Can you work these out from the model? Positions are in its coordinate system, mm. A direction names the side the tool comes from. Give positions to 0.01 mm unless a question says otherwise; leave off trailing zeros. Write each loop counter-clockwise with the first axis right and the second up, starting at its lowest first coordinate (ties: lowest second). Pieces come first, ordered by that corner, then holes.
from build123d import *

# Parameters (mm, degrees)
F0_R     = 1.55
F1_DEPTH = 5
F3_DEPTH = 165
F4_DEPTH = 25
F5_R     = 2.6
F6_DEPTH = 165.001


with BuildPart() as f1:
    # F0 (on Top) → F1 (new body)
    with BuildSketch(Plane.XY):
        Polygon((-10, -25), (10, -25), (10, -20), (10, 20), (10, 25), (-10, 25), (-10, 20), (-10, -20), align=None)
        with Locations((0, -10)):
            Circle(F0_R, mode=Mode.SUBTRACT)
        with Locations((0, 5)):
            Circle(F0_R, mode=Mode.SUBTRACT)
        Polygon((10, -20), (10, -25), (47.5, -55.5555555556), (47.5, -50.5555555556), align=None)
        Polygon((-47.5, -55.5555555556), (-10, -25), (-10, -20), (-47.5, -50.5555555556), align=None)
        Polygon((52.5, -59.6296296296), (47.5, -55.5555555556), (47.5, -95), (52.5, -95), align=None)
        Polygon((47.5, -50.5555555556), (47.5, -55.5555555556), (52.5, -59.6296296296), (52.5, -54.6296296296), align=None)
        Polygon((-52.5, -59.6296296296), (-47.5, -55.5555555556), (-47.5, -50.5555555556), (-52.5, -54.6296296296), align=None)
        Polygon((-47.5, -95), (-47.5, -55.5555555556), (-52.5, -59.6296296296), (-52.5, -95), align=None)
        Polygon((10, 25), (10, 20), (47.5, 50.5555555556), (47.5, 55.5555555556), align=None)
        Polygon((52.5, -54.6296296296), (52.5, -59.6296296296), (77.5, -80), (77.5, -75), align=None)
        Polygon((-47.5, 50.5555555556), (-10, 20), (-10, 25), (-47.5, 55.5555555556), align=None)
        Polygon((-77.5, -80), (-52.5, -59.6296296296), (-52.5, -54.6296296296), (-77.5, -75), align=None)
        Polygon((47.5, 55.5555555556), (47.5, 50.5555555556), (52.5, 54.6296296296), (52.5, 59.6296296296), align=None)
        Polygon((77.5, -75), (77.5, -80), (77.5, -95), (82.5, -95), (82.5, 95), (77.5, 95), (77.5, 80), (77.5, 75), align=None)
        Polygon((-52.5, 54.6296296296), (-47.5, 50.5555555556), (-47.5, 55.5555555556), (-52.5, 59.6296296296), align=None)
        Polygon((-77.5, -95), (-77.5, -80), (-77.5, -75), (-77.5, 75), (-77.5, 80), (-77.5, 95), (-82.5, 95), (-82.5, -95), align=None)
        Polygon((47.5, 95), (47.5, 55.5555555556), (52.5, 59.6296296296), (52.5, 95), align=None)
        Polygon((52.5, 59.6296296296), (52.5, 54.6296296296), (77.5, 75), (77.5, 80), align=None)
        Polygon((-52.5, 59.6296296296), (-47.5, 55.5555555556), (-47.5, 95), (-52.5, 95), align=None)
        Polygon((-77.5, 75), (-52.5, 54.6296296296), (-52.5, 59.6296296296), (-77.5, 80), align=None)
        Polygon((-52.5, -54.6296296296), (-47.5, -50.5555555556), (-47.5, 50.5555555556), (-52.5, 54.6296296296), align=None)
        Polygon((47.5, 50.5555555556), (47.5, -50.5555555556), (52.5, -54.6296296296), (52.5, 54.6296296296), align=None)
    extrude(amount=F1_DEPTH)

    # F2 (on face) → F3 (join, through all)
    with BuildSketch(Plane(origin=(-82.5, 0, 0), x_dir=(0, -1, 0), z_dir=(-1, 0, 0))):
        with BuildLine():
            Line((-95, 5), (-80, 5))
            ThreePointArc((-80, 5), (-87.5, 12.5), (-95, 5))
        make_face()
        with BuildLine():
            Line((80, 5), (95, 5))
            ThreePointArc((95, 5), (87.5, 12.5), (80, 5))
        make_face()
    extrude(amount=-F3_DEPTH)

    # F4 (cut): faces of the model
    f4_faces = [f1.faces().sort_by_distance(p)[0] for p in [
        (65, 87.5, 5),
        (0, 87.5, 5),
        (-65, 87.5, 5),
        (-65, -87.5, 5),
        (0, -87.5, 5),
        (65, -87.5, 5),
    ]]
    extrude(f4_faces, amount=-F4_DEPTH, mode=Mode.SUBTRACT)

    # F5 (on face) → F6 (cut, through all)
    with BuildSketch(Plane.YZ.offset(82.5)):
        with Locations((-87.5, 5)):
            Circle(F5_R)
        with Locations((87.5, 5)):
            Circle(F5_R)
    extrude(amount=-F6_DEPTH, mode=Mode.SUBTRACT)


solid = f1.part
(1) Imagine slicing it at D-D, the plane x = -23. Write out the boundary of the cut face in (y, z).
Returned:
outline: (-35.59, 0) - (-30.59, 0) - (-30.59, 5) - (-35.59, 5) - close; (30.59, 0) - (35.59, 0) - (35.59, 5) - (30.59, 5) - close
(2) If I drill on L1, parallel to Z at x = 81, y = -87; L2, parallel to X at y = 50, z = 2; L3, parallel to X at y = 47, z = 1, over which ranges is the centre line in solid material (lowest first)?
Returned:
L1: z = 0 to 2.45, 7.55 to 12.48
L2: x = -82.5 to -77.5, -52.5 to -47.5, -46.82 to -40.68, 40.68 to 46.82, 47.5 to 52.5, 77.5 to 82.5
L3: x = -82.5 to -77.5, -52.5 to -47.5, -43.14 to -37, 37 to 43.14, 47.5 to 52.5, 77.5 to 82.5
(3) For faces 4 (the face through (-64.82, 69.67, 2.46)), 5 (the face through (64.82, -69.67, 2.46)), 6 (the face through (77.5, 1, 2)), which set-ups out of +Z, -Z, +X, -X, +Y, -Y let a thin tool reach every point of the face, with its end or its side?
Returned:
face 4: +Z, -Z, +Y
face 5: +Z, -Z, -Y
face 6: +Z, -Z
(4) Will these pins go through, and if not, where does the flat tip stop? P1, Ø6, axis at x = -10.5, y = -32.5, coming from the -Z side; P2, Ø4, axis at x = 13.5, z = 2.5, coming from the -Y side; P3, Ø6, axis at y = 89, z = 3, coming from the +X side; P4, Ø6, axis at x = 29.5, z = 1.5, coming from the -Y side.
Returned:
P1: passes through
P2: stops at y = -29.48
P3: stops at x = 82.5
P4: stops at y = -43.33
(5) Imagine slicing it at A-A, the plane y = 87.5. Give the number of separate pieces and of enclosed holes in the cut face, plus the area to 3 significant figures.
Returned:
separate pieces: 8
enclosed holes: 0
area: 146 mm2
(6) Imagine slicing it at C-C, the plane y = -3.5. Write out the boundary of the cut face in (x, z).
Returned:
outline: (-82.5, 0) - (-77.5, 0) - (-77.5, 5) - (-82.5, 5) - close; (-52.5, 0) - (-47.5, 0) - (-47.5, 5) - (-52.5, 5) - close; (-10, 0) - (10, 0) - (10, 5) - (-10, 5) - close; (47.5, 0) - (52.5, 0) - (52.5, 5) - (47.5, 5) - close; (77.5, 0) - (82.5, 0) - (82.5, 5) - (77.5, 5) - close
(7) If we mould it in two halves opening along Z, with no side actions, what happens to faces 1 (the face through (-50, 84.9, 5.1)), 2 (the face through (-82.5, 1, 4)), 3 (the face through (80, 84.9, 5.1))? For each: +Z half, -Z half, draft (parallel to the pull), parting line (faces both ways), or undercut.
Returned:
face 1: undercut
face 2: draft
face 3: undercut
